```python
from build123d import *

# Parameters (mm, degrees)
F0_W     = 9.525
F0_H     = 79.375
F1_DEPTH = 31.75
F2_W     = 31.75
F2_H     = 25.4
F3_DEPTH = 12.7


with BuildPart() as f1:
    # F0 (on Front) → F1 (new body)
    with BuildSketch(Plane.XZ):
        with Locations((-4.7625, 39.6875)):
            Rectangle(F0_W, F0_H)
    extrude(amount=-F1_DEPTH)

    # F2 (on face) → F3 (join)
    with BuildSketch(Plane.YZ):
        with Locations((15.875, 66.675)):
            Rectangle(F2_W, F2_H)
    extrude(amount=F3_DEPTH)


solid = f1.part
```
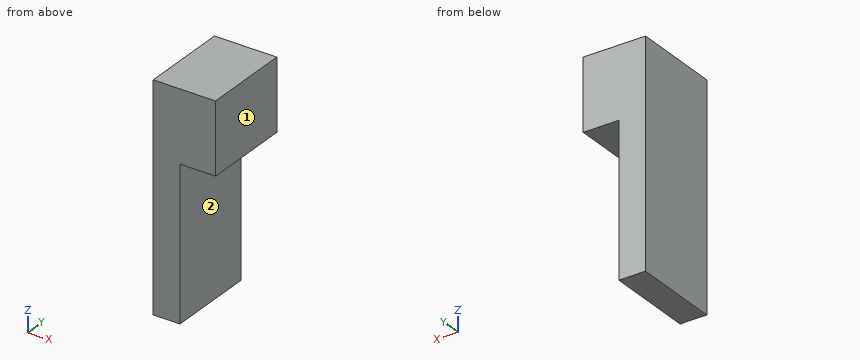
Verification items for the finished model (mm, model axes). Face numbers are marked on the shaded views. A direction names the side the tool comes from. Give positions to 0.01 mm unless a question says otherwise; leave off trailing zeros. Order: outer loops, then holes, each group sorted by start corner. A loop starts at its lowest first (then second) coordinate and runs counter-clockwise, first axis right, second up. Notation, with made-up numbers: M -12.75,18.5 L 12.25,18.5 A21 ccw 12.25,57.5 Z; hole C 47.25,-8 d10. An arc over 180 degrees is marked long. Answer in a Markdown table with one row per item. Add a question column.
Item 1: Scan lines: probe 1 along Z at (x, y) = (2.5, 12.5) (3 decimals); probe 2 along X at (y, z) = (27, 10.5) (3 decimals). Record each from-to range of solid material in increasing order. Write a range as from..to.
Item 2: Gauge pin test, flat ends, axial feed: pin 1 (10 mm diameter, centred on x = -3, y = 20.5, fed in from -Z); pin 2 (6 mm diameter, centred on y = 9.5, z = 17.5, fed in from +X); pin 3 (8 mm diameter, centred on x = 9.5, y = 8.5, fed in from -Z) (3 decimals). Record the tip position at first contact, or that the pin passes through.
Item 3: Section check C-C, the plane z = 18. Enter the section's corners in (x, y) (3 decimals).
Item 4: Section check B-B, the plane x = 2. Enter the section's corners in (y, z) (3 decimals).
Item 5: Tool access check on the marked faces 1 and 2. Record the directions out of +Z, -Z, +X, -X, +Y, -Y that give a thin tool (end or side, any length) a straight path to the whole face; none if there is none.
Item 6: Section check A-A, the plane y = 7.5. Enter the section's corners in (x, z) (3 decimals).
Filled sheet:
| question | item | result |
|---|---|---|
| 1 | probe 1 | z = 53.975..79.375 |
| 1 | probe 2 | x = -9.525..0 |
| 2 | pin 1 | stops at z = 0 |
| 2 | pin 2 | stops at x = 0 |
| 2 | pin 3 | stops at z = 53.975 |
| 3 | outline | M -9.525,0 L 0,0 L 0,31.75 L -9.525,31.75 Z |
| 4 | outline | M 0,53.975 L 31.75,53.975 L 31.75,79.375 L 0,79.375 Z |
| 5 | face 1 | +Z, -Z, +X, +Y, -Y |
| 5 | face 2 | -Z, +X, +Y, -Y |
| 6 | outline | M -9.525,0 L 0,0 L 0,53.975 L 12.7,53.975 L 12.7,79.375 L -9.525,79.375 Z |
